```python
from build123d import *

# Parameters (mm, degrees)
SKETCH1_W           = 146
SKETCH1_H           = 37
BOSS_EXTRUDE1_DEPTH = 2
BOSS_EXTRUDE2_DEPTH = 4


with BuildPart() as part:
    # Sketch1 → Boss-Extrude1 (new body)
    with BuildSketch(Plane.XY):
        with Locations((75, 18.5)):
            Rectangle(SKETCH1_W, SKETCH1_H)
    extrude(amount=BOSS_EXTRUDE1_DEPTH)

    # Sketch1<4> → Boss-Extrude2 (add)
    with BuildSketch(Plane.XY):
        Polygon((2, 0), (2, 37), (148, 37), (148, 0), (150, 0), (150, 40), (0, 40), (0, 0), align=None)
    extrude(amount=BOSS_EXTRUDE2_DEPTH)

    # Chamfer1
    # the kernel refuses this chamfer: 3, 1.732050808 mm, written as the material it takes off along each edge
    with BuildSketch(Plane(origin=(148, 37, 4), x_dir=(-0.05789386240267211, 0, -0.9983227437537925), z_dir=(0, -1, 0)), Plane(origin=(2, 0, 4), x_dir=(0.05789386240267088, 0, -0.9983227437537927), z_dir=(0, 1, 0))) as chamfer1_piece_1:
        with BuildLine():
            Line((1.795061586, 0), (-0.239597459, 3.095243342))
            Line((-0.239597459, 3.095243342), (-0.299496823, 3.091769711))
            ThreePointArc((-0.299496823, 3.091769711), (-0.149748412, 1.545884855), (-0.059899365, -0.003473632))
            Line((-0.059899365, -0.003473632), (0.003473632, -0.059899365))
            ThreePointArc((0.003473632, -0.059899365), (0.897996171, -0.008024993), (1.798535218, -0.059899365))
            Line((1.798535218, -0.059899365), (1.795061586, 0))
        make_face()
    extrude(amount=37, mode=Mode.SUBTRACT)
    with BuildSketch(Plane(origin=(2, 37, 4), x_dir=(0, -0.05789386240267211, -0.9983227437537925), z_dir=(1, 0, 0))) as chamfer1_piece_2:
        with BuildLine():
            Line((1.795061586, 0), (-0.239597459, 3.095243342))
            Line((-0.239597459, 3.095243342), (-0.299496823, 3.091769711))
            ThreePointArc((-0.299496823, 3.091769711), (-0.149748412, 1.545884855), (-0.059899365, -0.003473632))
            Line((-0.059899365, -0.003473632), (0.003473632, -0.059899365))
            ThreePointArc((0.003473632, -0.059899365), (0.897996171, -0.008024993), (1.798535218, -0.059899365))
            Line((1.798535218, -0.059899365), (1.795061586, 0))
        make_face()
    extrude(amount=146, mode=Mode.SUBTRACT)
    with BuildSketch(Plane(origin=(148, 44.761257264, 4), x_dir=(-0.05789386240267211, 0, -0.9983227437537925), z_dir=(0, -1, 0))) as chamfer1_piece_3a_section:
        with BuildLine():
            Line((1.795061586, 0), (-0.239597459, 3.095243342))
            Line((-0.239597459, 3.095243342), (-0.299496823, 3.091769711))
            ThreePointArc((-0.299496823, 3.091769711), (-0.149748412, 1.545884855), (-0.059899365, -0.003473632))
            Line((-0.059899365, -0.003473632), (0.003473632, -0.059899365))
            ThreePointArc((0.003473632, -0.059899365), (0.897996171, -0.008024993), (1.798535218, -0.059899365))
            Line((1.798535218, -0.059899365), (1.795061586, 0))
        make_face()
    chamfer1_piece_3a = extrude(amount=44.761257264, mode=Mode.PRIVATE)
    chamfer1_piece_3a = split(chamfer1_piece_3a, bisect_by=Plane(origin=(149.006146815, 37, 3.444583449), z_dir=(0, 1, 0)), keep=Keep.TOP, mode=Mode.PRIVATE)
    with BuildSketch(Plane(origin=(2, 37, 4), x_dir=(0, -0.05789386240267211, -0.9983227437537925), z_dir=(1, 0, 0))) as chamfer1_piece_3b_section:
        with BuildLine():
            Line((1.795061586, 0), (-0.239597459, 3.095243342))
            Line((-0.239597459, 3.095243342), (-0.299496823, 3.091769711))
            ThreePointArc((-0.299496823, 3.091769711), (-0.149748412, 1.545884855), (-0.059899365, -0.003473632))
            Line((-0.059899365, -0.003473632), (0.003473632, -0.059899365))
            ThreePointArc((0.003473632, -0.059899365), (0.897996171, -0.008024993), (1.798535218, -0.059899365))
            Line((1.798535218, -0.059899365), (1.795061586, 0))
        make_face()
    chamfer1_piece_3b = extrude(amount=153.761257264, mode=Mode.PRIVATE)
    chamfer1_piece_3b = split(chamfer1_piece_3b, bisect_by=Plane(origin=(148, 38.006146815, 3.444583449), z_dir=(1, 0, 0)), keep=Keep.TOP, mode=Mode.PRIVATE)
    chamfer1_piece_3 = chamfer1_piece_3a & chamfer1_piece_3b
    add(chamfer1_piece_3, mode=Mode.SUBTRACT)
    with BuildSketch(Plane(origin=(-5.761257264, 37, 4), x_dir=(0, -0.05789386240267211, -0.9983227437537925), z_dir=(1, 0, 0))) as chamfer1_piece_4a_section:
        with BuildLine():
            Line((1.795061586, 0), (-0.239597459, 3.095243342))
            Line((-0.239597459, 3.095243342), (-0.299496823, 3.091769711))
            ThreePointArc((-0.299496823, 3.091769711), (-0.149748412, 1.545884855), (-0.059899365, -0.003473632))
            Line((-0.059899365, -0.003473632), (0.003473632, -0.059899365))
            ThreePointArc((0.003473632, -0.059899365), (0.897996171, -0.008024993), (1.798535218, -0.059899365))
            Line((1.798535218, -0.059899365), (1.795061586, 0))
        make_face()
    chamfer1_piece_4a = extrude(amount=153.761257264, mode=Mode.PRIVATE)
    chamfer1_piece_4a = split(chamfer1_piece_4a, bisect_by=Plane(origin=(2, 38.006146815, 3.444583449), z_dir=(-1, 0, 0)), keep=Keep.TOP, mode=Mode.PRIVATE)
    with BuildSketch(Plane(origin=(2, 0, 4), x_dir=(0.05789386240267088, 0, -0.9983227437537927), z_dir=(0, 1, 0))) as chamfer1_piece_4b_section:
        with BuildLine():
            Line((1.795061586, 0), (-0.239597459, 3.095243342))
            Line((-0.239597459, 3.095243342), (-0.299496823, 3.091769711))
            ThreePointArc((-0.299496823, 3.091769711), (-0.149748412, 1.545884855), (-0.059899365, -0.003473632))
            Line((-0.059899365, -0.003473632), (0.003473632, -0.059899365))
            ThreePointArc((0.003473632, -0.059899365), (0.897996171, -0.008024993), (1.798535218, -0.059899365))
            Line((1.798535218, -0.059899365), (1.795061586, 0))
        make_face()
    chamfer1_piece_4b = extrude(amount=44.761257264, mode=Mode.PRIVATE)
    chamfer1_piece_4b = split(chamfer1_piece_4b, bisect_by=Plane(origin=(0.993853185, 37, 3.444583449), z_dir=(0, 1, 0)), keep=Keep.TOP, mode=Mode.PRIVATE)
    chamfer1_piece_4 = chamfer1_piece_4a & chamfer1_piece_4b
    add(chamfer1_piece_4, mode=Mode.SUBTRACT)


solid = part.part
```
Can you work these out from the model? Positions are in its coordinate system, mm. A direction names the side the tool comes from. Coordinates: 2 decimals unless noted, no trailing zeros. Loops run counter-clockwise (first coordinate to the right, second up) from the corner with the lowest first, then second, coordinate; pieces in that order, holes last. Notation, with made-up numbers: (54.25, 25) -> (81.25, 25) arc R20 ccw to (81.25, 55) -> close; hole circle Ø8 at (20, 21). An arc over 180 degrees is marked (long way). Answer as a JSON object with one key per item and string values.
1) Thinking about a two-plate mould opening in X: for faces 1 (the face through (0, 20, 2)), 2 (the face through (73.95, 38.479, 3.122)), 3 (the face through (76, 40, 2)), which applies, pulls with the +X half, pulls with the -X half, needs draft (parallel to the pull), parting line crosses it, or undercut?
Results:
{"face 1": "pulls with the -X half", "face 2": "undercut", "face 3": "needs draft"}
2) If I drill on line 1 (Z direction, x = 110.5, y = 4.5); line 2 (Y direction, x = 67.5, z = 2.2); line 3 (X direction, y = 24.5, z = 2.4), over which ranges is the centre line in solid material (lowest first)?
Results:
{"line 1": "z = 0 to 2", "line 2": "y = 37 to 40", "line 3": "x = 0 to 1.77, 148.23 to 150"}
3) For faces 4 (the face through (74, 19, 2)), 5 (the face through (74, 20, 0)), which set-ups out of +Z, -Z, +X, -X, +Y, -Y let a thin tool reach every point of the face, with its end or its side?
Results:
{"face 4": "+Z, -Y", "face 5": "-Z, +X, -X, +Y, -Y"}
4) Imagine slicing it at A-A (y = 26). Please give me the cut outline in (x, z), then the cut area to 3 significant figures.
Results:
{"outline": "(0, 0) -> (150, 0) -> (150, 3.42) -> (148, 2.27) -> (148, 2) -> (2, 2) -> (2, 2.27) -> (0, 3.42) -> close", "area": "303 mm^2"}
5) For P1, Ø5, axis at x = 53, y = 17, coming from the +Z side, with a flat end and sliding along its axis, tell me the tip position at first contact or that it passes through.
Results:
{"P1": "stops at z = 2"}
6) Imagine slicing it at B-B (x = 86.5). Please give me the cut outline in (y, z), then the cut area to 3 significant figures.
Results:
{"outline": "(0, 0) -> (40, 0) -> (40, 4) -> (37, 2.27) -> (37, 2) -> (0, 2) -> close", "area": "83.4 mm^2"}
